```python
from build123d import *

# Parameters (mm, degrees)
SKETCH1_R           = 3.5
BOSS_EXTRUDE1_DEPTH = 5.5
SKETCH2_R           = 2.75
CUT_EXTRUDE1_DEPTH  = 5.5
CUT_EXTRUDE1_TAPER  = 12
CUT_EXTRUDE2_DEPTH  = 5.5
CIRPATTERN1_COUNT   = 10
SKETCH4_R           = 2.75
CUT_EXTRUDE3_DEPTH  = 5
CUT_EXTRUDE3_TAPER  = 9
SKETCH5_R           = 4
SKETCH5_R_2         = 3.5
SKETCH5_R_3         = 2.75
BOSS_EXTRUDE2_DEPTH = 1


with BuildPart() as part:
    # Sketch1 → Boss-Extrude1 (new body)
    with BuildSketch(Plane(origin=(0, 0, 0), x_dir=(1, 0, 0), z_dir=(0, 1, 0))):
        Circle(SKETCH1_R)
    extrude(amount=BOSS_EXTRUDE1_DEPTH)

    # Sketch2 → Cut-Extrude1 (cut)
    with BuildSketch(Plane.XZ):
        Circle(SKETCH2_R)
    extrude(amount=-CUT_EXTRUDE1_DEPTH, taper=CUT_EXTRUDE1_TAPER, mode=Mode.SUBTRACT)

    # Sketch3 → Cut-Extrude2 (cut)
    with BuildSketch(Plane(origin=(0, 0, 0), x_dir=(0, 0, -1), z_dir=(1, 0, 0))):
        Polygon((-0.5, 5.5), (-0.35, 4.3), (0, 1.5), (0.35, 4.3), (0.5, 5.5), align=None)
    cut_extrude2 = extrude(amount=-CUT_EXTRUDE2_DEPTH, mode=Mode.SUBTRACT)

    # CirPattern1: Cut-Extrude2 ×10 about axis
    cirpattern1_axis = Axis((0, 5.5, 0), (0, -1, 0))
    for i in range(1, CIRPATTERN1_COUNT):
        add(cut_extrude2.rotate(cirpattern1_axis, i * 360 / CIRPATTERN1_COUNT), mode=Mode.SUBTRACT)

    # Sketch4 → Cut-Extrude3 (cut)
    with BuildSketch(Plane.XZ):
        Circle(SKETCH4_R)
    extrude(amount=-CUT_EXTRUDE3_DEPTH, taper=CUT_EXTRUDE3_TAPER, mode=Mode.SUBTRACT)

    # Sketch5 → Boss-Extrude2 (add)
    with BuildSketch(Plane.XZ):
        Circle(SKETCH5_R)
        Circle(SKETCH5_R_2, mode=Mode.SUBTRACT)
        Circle(SKETCH5_R_2)
        Circle(SKETCH5_R_3, mode=Mode.SUBTRACT)
    extrude(amount=BOSS_EXTRUDE2_DEPTH)


solid = part.part
```
Can you work these out from the model? Positions are in its coordinate system, mm. Coordinates: 2 decimals unless noted, no trailing zeros. Loops run counter-clockwise (first coordinate to the right, second up) from the corner with the lowest first, then second, coordinate; pieces in that order, holes last. Notation, with made-up numbers: (-22.75, 38.25) - (-1.75, 38.25) arc R27 ccw to (-1.75, 71.25) - close; hole circle Ø11 at (45.25, -30.75). An arc over 180 degrees is marked (long way). Use a Markdown table: item, result.
Item 1: If I drill on probe 1 along Z at (x, y) = (0, -0.7); probe 2 along Z at (x, y) = (0, 5.25); probe 3 along Z at (x, y) = (-2, 3.25), over which ranges is the centre line in solid material (lowest first)? Write a range as from..to.
Numbers:
| item | result |
|---|---|
| probe 1 | z = -4..-2.75, 2.75..4 |
| probe 2 | z = -3.5..-1.63, 1.63..3.5 |
| probe 3 | z = -2.87..-1.72, -1.18..-1, 1..1.18, 1.72..2.87 |
Item 2: Will these pins go through, and if not, where does the flat tip stop? pin 1 (2 mm diameter, centred on x = -2.5, y = -0.5, fed in from -Z); pin 2 (3 mm diameter, centred on x = -2, y = 3, fed in from +Z).
Numbers:
| item | result |
|---|---|
| pin 1 | stops at z = -3.71 |
| pin 2 | stops at z = 3.46 |
Item 3: I want a section at A-A on y = 0.75. Please give me the cut outline in (x, z).
Numbers:
| item | result |
|---|---|
| outline | circle Ø7 at (0, 0); hole circle Ø5.26 at (0, 0) |
Item 4: We'd pull the mould along Z, two halves only. Please class faces 1 (the face through (3, 5.5, 1)), 2 (the face through (1.073, 3.472, -2.505)), 3 (the face through (3.34, 2.71, -1.05)): released by +Z, released by -Z, zero draft, split by the parting line, or undercut.
Numbers:
| item | result |
|---|---|
| face 1 | zero draft |
| face 2 | undercut |
| face 3 | split by the parting line |
Item 5: I want a section at B-B on y = 2. Give the number of separate pieces and of enclosed holes in the cut face, and give its area (3 significant figures).
Numbers:
| item | result |
|---|---|
| separate pieces | 10 |
| enclosed holes | 0 |
| area | 18.6 mm2 |
